Geometry: final body of the model. Coordinates: model frame, mm. Face numbers are marked on the shaded views. A direction names the side the tool comes from. Coordinates: 2 decimals unless noted, no trailing zeros. Order: outer loops, then holes, each group sorted by start corner. A loop starts at its lowest first (then second) coordinate and runs counter-clockwise, first axis right, second up. Notation, with made-up numbers: M 19,15 L 55,15 A26 ccw 55,38 Z; hole C 69,42 d4. An arc over 180 degrees is marked long. Use CSV: the item, a comma, the result in double quotes. Start each with the question number.
Q1. First-contact query: P1, Ø1, axis at x = -6.5, z = 15.5, coming from the -Y side; P2, Ø6, axis at x = 9.5, z = 15.5, coming from the +Y side; P3, Ø9, axis at y = -25, z = 0, coming from the +X side; P4, Ø10, axis at x = -7, z = 11.5, coming from the +Y side. Flat tips, straight axial feed; report the tip coordinate or a pass-through.
Q2. Section query B-B, the plane y = -29. Output: boundary loops of the cut face in (x, z), and give its area (3 significant figures).
Q3. Ray query, probe 1 along X at (y, z) = (-25, 6); probe 2 along Z at (x, y) = (-11.75, -25); probe 3 along X at (y, z) = (-2, -10). Return the intervals inside material, ascending.
Q4. Mould query, pull axis X, two halves, no side actions, for the marked faces 1, 2 and 3. Classes: +X half, -X half, draft (parallel to the pull), parting line (faces both ways), or undercut.
Q5. Section query D-D, the plane z = 3.5. Output: boundary loops of the cut face in (x, y), and give its area (3 significant figures).
Q6. Access query for the marked faces 4, 5 and 6. Directions: +Z, -Z, +X, -X, +Y, -Y. A direction counts if a zero-diameter tool reaches every point of the face in a straight line with its end or side. Return the directions, or none.
Q7. Section query A-A, the plane y = -33. Output: boundary loops of the cut face in (x, z).
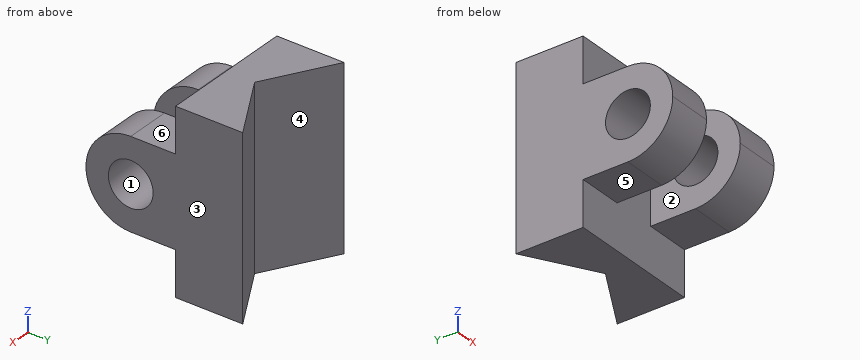
from build123d import *

# Parameters (mm, degrees)
F0_W     = 30
F0_H     = 40
F1_DEPTH = 15
F2_W     = 10
F2_H     = 20
F3_DEPTH = 20
F4_R     = 5
F5_DEPTH = 30.001
F6_R     = 9.99999
F8_DEPTH = 40.001


# Not quite as in the source:
# - a fillet or chamfer is up to 0.001 mm smaller than in the source, because OpenCascade refuses the exact size


with BuildPart() as f1:
    # F0 (on Front) → F1 (new body)
    with BuildSketch(Plane.XZ):
        Rectangle(F0_W, F0_H)
    extrude(amount=F1_DEPTH)

    # F2 (on face) → F3 (join)
    with BuildSketch(Plane.XZ.offset(15)):
        with Locations((-10, 0)):
            Rectangle(F2_W, F2_H)
        with Locations((10, 0)):
            Rectangle(F2_W, F2_H)
    extrude(amount=F3_DEPTH)

    # F4 (on face) → F5 (cut, through all)
    with BuildSketch(Plane.YZ.offset(15)):
        with Locations((-25, 0)):
            Circle(F4_R)
    extrude(amount=-F5_DEPTH, mode=Mode.SUBTRACT)

    # F6 (radius 10 in the source; OpenCascade refuses exactly that, so slightly less here)
    f6_edges = [f1.edges().sort_by_distance(p)[0] for p in [
        (10, -35, 10),
        (-10, -35, 10),
        (-10, -35, -10),
        (10, -35, -10),
    ]]
    fillet(f6_edges, radius=F6_R)

    # F7 (on face) → F8 (cut, through all)
    with BuildSketch(Plane.XY.offset(20)):
        Polygon((15, 0), (-15, 0), (0, -8.6602540378), align=None)
    extrude(amount=-F8_DEPTH, mode=Mode.SUBTRACT)


solid = f1.part
Responses:
1,P1,"stops at y = -15"
1,P2,"stops at y = -1.44"
1,P3,"passes through"
1,P4,"stops at y = -1.73"
2,outline,"M -15,-9.17 L -5,-9.17 L -5,-3 L -15,-3 Z; M -15,3 L -5,3 L -5,9.17 L -15,9.17 Z; M 5,-9.17 L 15,-9.17 L 15,-3 L 5,-3 Z; M 5,3 L 15,3 L 15,9.17 L 5,9.17 Z"
2,area,"247 mm²"
3,probe 1,"x = -15 to -5, 5 to 15"
3,probe 2,"z = -10 to -5, 5 to 10"
3,probe 3,"x = -15 to -11.54, 11.54 to 15"
4,face 1,"draft"
4,face 2,"undercut"
4,face 3,"+X half"
5,outline,"M -15,-34.37 L -5,-34.37 L -5,-28.57 L -15,-28.57 Z; M -15,-21.43 L -5,-21.43 L -5,-15 L 5,-15 L 5,-21.43 L 15,-21.43 L 15,0 L 0,-8.66 L -15,0 Z; M 5,-34.37 L 15,-34.37 L 15,-28.57 L 5,-28.57 Z"
5,area,"565 mm²"
6,face 4,"+Z, -Z, +Y"
6,face 5,"-Z, +X, -X, -Y"
6,face 6,"+Z, +X, -X, -Y"
7,outline,"M -15,-6 L -5,-6 L -5,6 L -15,6 Z; M 5,-6 L 15,-6 L 15,6 L 5,6 Z"
